Autodesk Inventor part; units mm, degrees
ref_plane "YZ Plane" through (0, 0, 0) normal (1, 0, 0) x (0, 1, 0)
ref_plane "XZ Plane" through (0, 0, 0) normal (0, 1, 0) x (-1, 0, 0)
ref_plane "XY Plane" through (0, 0, 0) normal (0, 0, 1) x (1, 0, 0)
sketch "Skizze1" plane through (0, 0, 0) normal (0, 0, 1) x (1, 0, 0)
  line L0 (0, 5) -> (0, 95)
  line L1 (5, 100) -> (45, 100)
  line L2 (50, 95) -> (50, 5)
  arc A0 (5, 100) -> (0, 95) centre (5, 95) ccw
  arc A1 (50, 95) -> (45, 100) centre (45, 95) ccw
  arc A2 (45, 0) -> (50, 5) centre (45, 5) ccw
  arc A3 (0, 5) -> (5, 0) centre (5, 5) ccw
  line L3 (10, 0) -> (10, -11)
  line L4 (10, -11) -> (20, -11)
  line L5 (20, -11) -> (20, 0)
  line L6 (30, 0) -> (30, -11)
  line L7 (30, -11) -> (40, -11)
  line L8 (40, -11) -> (40, 0)
  line L9 (5, 0) -> (10, 0)
  line L10 (20, 0) -> (30, 0)
  line L11 (40, 0) -> (45, 0)
  line L12 (5, 40) -> (45, 40)
  arc A4 (6.0261, 45.8191) -> (5, 40) centre (5, 43) ccw
  arc A5 (45, 40) -> (46.0261, 45.8191) centre (45, 43) ccw
  arc A6 (46.0261, 45.8191) -> (41.3553, 51.3855) centre (42.4089, 47.5268) ccw
  arc A7 (13.45, 52.0485) -> (6.0261, 45.8191) centre (10.5305, 47.9894) ccw
  arc A8 (31.0213, 55.1468) -> (13.45, 52.0485) centre (22.442, 52.4271) ccw
  line L13 (5, 40) -> (6.0261, 45.8191) construction
  line L14 (6.0261, 45.8191) -> (13.45, 52.0485) construction
  line L15 (13.45, 52.0485) -> (31.0213, 55.1468) construction
  line L16 (41.3553, 51.3855) -> (46.0261, 45.8191) construction
  line L17 (45, 40) -> (46.0261, 45.8191) construction
  arc A9 (41.3553, 51.3855) -> (31.0213, 55.1468) centre (36.2306, 53.3825) ccw
  line L18 (31.0213, 55.1468) -> (41.3553, 51.3855) construction
  point P0 (0, 0)
  point P1 (25, 40)
  point P2 (25, 0)
  dimension "d1" = 50
  dimension "d3" = 5
  dimension "d4" = 11
  dimension "d5" = 10
  dimension "d6" = 100
  dimension "d15" = 40
  dimension "d24" = 40
  dimension "d28" = 3
  dimension "d29" = 3
  dimension "d30" = 100
  dimension "d31" = 4
  dimension "d32" = 130
  dimension "d33" = 80
  dimension "d34" = 140
  dimension "d35" = 5
  dimension "d36" = 9
  dimension "d37" = 5.5
  dimension "d38" = 150
  dimension "d39" = 150
  dimension "d40" = 12.0485
  dimension "d41" = 11.3855
extrude "Extrusion1" add sketch "Skizze1" along normal blind 3
properties part number "Scheibe" material "Glas"
Check sheet for the modelled part. Datum: model origin and axes. Units: mm. A direction names the side the tool comes from. Give positions to 0.01 mm unless a question says otherwise; leave off trailing zeros. Write each loop counter-clockwise with the first axis right and the second up, starting at its lowest first coordinate (ties: lowest second). Pieces come first, ordered by that corner, then holes. Notation, with made-up numbers: (51, 72.5) -> (58, 72.5) arc R29 cw to (58, 110.5) -> close; hole circle Ø10 at (-32, 11). An arc over 180 degrees is marked (long way). Write item = value, one per line.
Item 1: Release check for a two-part mould opening along X. For faces 1 (the flat face through (30, 58, 3)), 2 (the cylindrical face through (1, 98, 1)), 3 (the cylindrical face through (45.43, 50.15, 1.48)) record: +X half, -X half, draft (parallel to the pull), parting line (faces both ways), or undercut.
Output:
face_1 = draft
face_2 = -X half
face_3 = undercut
Item 2: Sectioned sample at A-A on y = -4. Record the boundary of the cut face in (x, z).
Output:
outline = (10, 0) -> (20, 0) -> (20, 3) -> (10, 3) -> close; (30, 0) -> (40, 0) -> (40, 3) -> (30, 3) -> close
Item 3: Tool access check on faces 4 (the flat face through (40, -6, 1)), 5 (the flat face through (35, -11, 1)), 6 (the flat face through (10, -5, 1)), 7 (the flat face through (50, 51, 1)), 8 (the flat face through (30, -5, 1)). Record the directions out of +Z, -Z, +X, -X, +Y, -Y that give a thin tool (end or side, any length) a straight path to the whole face; none if there is none.
Output:
face_4 = +Z, -Z, +X, -Y
face_5 = +Z, -Z, +X, -X, -Y
face_6 = +Z, -Z, -X, -Y
face_7 = +Z, -Z, +X, +Y, -Y
face_8 = +Z, -Z, -Y
Item 4: Sectioned sample at B-B on x = 24. Record the boundary of the cut face in (y, z).
Output:
outline = (0, 0) -> (40, 0) -> (40, 3) -> (0, 3) -> close; (61.29, 0) -> (100, 0) -> (100, 3) -> (61.29, 3) -> close
Item 5: Gauge pin test, flat ends, axial feed: pin 1 (5 mm diameter, centred on x = 5, y = 43, fed in from -Z); pin 2 (0.9 mm diameter, centred on x = 42.5, z = 1, fed in from -Y); pin 3 (0.9 mm diameter, centred on y = -4.5, z = 1.5, fed in from +X); pin 4 (0.9 mm diameter, centred on y = -7, z = 1, fed in from -X). Record the tip position at first contact, or that the pin passes through.
Output:
pin_1 = through
pin_2 = 0
pin_3 = 40
pin_4 = 10
Item 6: Scan lines: probe 1 along Y at (x, z) = (42, 2.8); probe 2 along Y at (x, z) = (17, 1.7); probe 3 along X at (y, z) = (52.5, 1.65). Record each from-to range of solid material in increasing order. Write a range as from..to.
Output:
probe_1 = 0..40, 51.51..100
probe_2 = -11..40, 59.6..100
probe_3 = 0..8.37, 12.69..13.44, 41.66..50
Item 7: Sectioned sample at C-C on z = 0.7. Record the boundary of the cut face in (x, y), and give its area (3 significant figures).
Output:
outline = (0, 5) arc R5 ccw to (5, 0) -> (10, 0) -> (10, -11) -> (20, -11) -> (20, 0) -> (30, 0) -> (30, -11) -> (40, -11) -> (40, 0) -> (45, 0) arc R5 ccw to (50, 5) -> (50, 95) arc R5 ccw to (45, 100) -> (5, 100) arc R5 ccw to (0, 95) -> close; hole (5, 40) -> (45, 40) arc R3 ccw to (46.03, 45.82) arc R4 ccw to (41.36, 51.39) arc R5.5 ccw (long way) to (31.02, 55.15) arc R9 ccw to (13.45, 52.05) arc R5 ccw to (6.03, 45.82) arc R3 ccw (long way) to start
area = 4,490 mm^2
